```python
from build123d import *

# Parameters (mm, degrees)
SKETCH1_W           = 56
SKETCH1_H           = 56
BOSS_EXTRUDE1_DEPTH = 25
SKETCH2_W           = 53.2
SKETCH2_H           = 53.2
CUT_EXTRUDE1_DEPTH  = 22
SKETCH3_R           = 1.7
CUT_EXTRUDE2_DEPTH  = 1.4
SKETCH4_W           = 25.2
SKETCH4_H           = 27.2
CUT_EXTRUDE3_DEPTH  = 3
SKETCH5_W           = 4
SKETCH5_H           = 4
BOSS_EXTRUDE2_DEPTH = 3
SKETCH6_W           = 8
SKETCH6_H           = 8
BOSS_EXTRUDE3_DEPTH = 5
SKETCH7_R           = 2
CUT_EXTRUDE4_DEPTH  = 8
BOSS_EXTRUDE4_DEPTH = 3
FILLET1_R           = 1
CHAMFER1_SIZE       = 1.35
FILL_PATTERN1_DEPTH = 3


# Read off the part's stored shape, not the designer's step: Fill Pattern1
with BuildPart() as part:
    # Sketch1 → Boss-Extrude1 (new body)
    with BuildSketch(Plane(origin=(0, 0, 0), x_dir=(1, 0, 0), z_dir=(0, 1, 0))):
        Rectangle(SKETCH1_W, SKETCH1_H)
    extrude(amount=BOSS_EXTRUDE1_DEPTH)

    # Sketch2 → Cut-Extrude1 (cut)
    with BuildSketch(Plane(origin=(0, 25, 0), x_dir=(1, 0, 0), z_dir=(0, 1, 0))):
        Rectangle(SKETCH2_W, SKETCH2_H)
    extrude(amount=-CUT_EXTRUDE1_DEPTH, mode=Mode.SUBTRACT)

    # Sketch3 → Cut-Extrude2 (cut)
    with BuildSketch(Plane.XY.offset(28)):
        with Locations((0, 21.6)):
            Circle(SKETCH3_R)
    extrude(amount=-CUT_EXTRUDE2_DEPTH, mode=Mode.SUBTRACT)

    # Sketch4 → Cut-Extrude3 (cut)
    with BuildSketch(Plane.XZ):
        with Locations((0, 8.1)):
            Rectangle(SKETCH4_W, SKETCH4_H)
    extrude(amount=-CUT_EXTRUDE3_DEPTH, mode=Mode.SUBTRACT)

    # Sketch5 → Boss-Extrude2 (add)
    with BuildSketch(Plane.XZ):
        with Locations((-10.6, 19.7)):
            Rectangle(SKETCH5_W, SKETCH5_H)
        with Locations((10.6, 19.7)):
            Rectangle(SKETCH5_W, SKETCH5_H)
        with Locations((10.6, -3.5)):
            Rectangle(SKETCH5_W, SKETCH5_H)
        with Locations((-10.6, -3.5)):
            Rectangle(SKETCH5_W, SKETCH5_H)
    extrude(amount=-BOSS_EXTRUDE2_DEPTH)

    # Sketch6 → Boss-Extrude3 (add)
    with BuildSketch(Plane(origin=(0, 3, 0), x_dir=(1, 0, 0), z_dir=(0, 1, 0))):
        with Locations((16.6, -19.7)):
            Rectangle(SKETCH6_W, SKETCH6_H)
        with Locations((-16.6, -19.7)):
            Rectangle(SKETCH6_W, SKETCH6_H)
        Polygon((12.6, -0.5), (20.6, -0.5), (22.6, -0.5), (22.6, 9.5), (12.6, 9.5), (12.6, 7.5), align=None)
        Polygon((-12.6, -0.5), (-20.6, -0.5), (-22.6, -0.5), (-22.6, 9.5), (-12.6, 9.5), (-12.6, 7.5), align=None)
    extrude(amount=BOSS_EXTRUDE3_DEPTH)

    # Sketch7 → Cut-Extrude4 (cut)
    with BuildSketch(Plane(origin=(0, 8, 0), x_dir=(1, 0, 0), z_dir=(0, 1, 0))):
        with Locations(Location((16.6, -19.7, 0), (0, 0, 270))):
            Circle(SKETCH7_R)
        with Locations(Location((-16.6, -19.7, 0), (0, 0, 270))):
            Circle(SKETCH7_R)
        with Locations(Location((16.6, 3.5, 0), (0, 0, 270))):
            Circle(SKETCH7_R)
        with Locations(Location((-16.6, 3.5, 0), (0, 0, 270))):
            Circle(SKETCH7_R)
    extrude(amount=-CUT_EXTRUDE4_DEPTH, mode=Mode.SUBTRACT)

    # Sketch9 → Boss-Extrude4 (add)
    with BuildSketch(Plane(origin=(0, 8, 0), x_dir=(1, 0, 0), z_dir=(0, 1, 0))):
        Polygon((-22.6, -0.5), (-22.6, 9.5), (-12.6, 9.5), (-12.6, 7.65), (-20.75, 7.65), (-20.75, -0.5), align=None)
        Polygon((12.6, 9.5), (22.6, 9.5), (22.6, -0.5), (20.75, -0.5), (20.75, 7.65), (12.6, 7.65), align=None)
    extrude(amount=BOSS_EXTRUDE4_DEPTH)

    # Fillet1
    fillet1_edges = [part.edges().sort_by_distance(p)[0] for p in [
        (0, 0, 28),
        (-28, 0, 0),
        (0, 0, -28),
        (28, 0, 0),
        (28, 12.5, 28),
        (-28, 12.5, 28),
        (-28, 12.5, -28),
        (28, 12.5, -28),
    ]]
    fillet(fillet1_edges, radius=FILLET1_R)

    # Chamfer1
    chamfer1_edges = [part.edges().sort_by_distance(p)[0] for p in [
        (-1.7, 21.6, 28),
    ]]
    chamfer(chamfer1_edges, length=CHAMFER1_SIZE)

    # Fill Pattern1 outline → Fill Pattern1 (cut)
    with BuildSketch(Plane(origin=(0, 0, 0), x_dir=(1, 0, 0), z_dir=(0, 1, 0))):
        Polygon((22.516660498, 17), (24.248711306, 20), (22.516660498, 23), (19.052558883, 23), (17.320508076, 20), (19.052558883, 17), align=None)
        Polygon((8.660254038, 23), (5.196152423, 23), (3.464101615, 20), (5.196152423, 17), (8.660254038, 17), (10.392304845, 20), align=None)
        Polygon((-5.196152423, 23), (-8.660254038, 23), (-10.392304845, 20), (-8.660254038, 17), (-5.196152423, 17), (-3.464101615, 20), align=None)
        Polygon((-19.052558883, 23), (-22.516660498, 23), (-24.248711306, 20), (-22.516660498, 17), (-19.052558883, 17), (-17.320508076, 20), align=None)
        Polygon((1.732050808, 13), (3.464101615, 16), (1.732050808, 19), (-1.732050808, 19), (-3.464101615, 16), (-1.732050808, 13), align=None)
        Polygon((-12.124355653, 19), (-15.588457268, 19), (-17.320508076, 16), (-15.588457268, 13), (-12.124355653, 13), (-10.392304845, 16), align=None)
        Polygon((15.588457268, 19), (12.124355653, 19), (10.392304845, 16), (12.124355653, 13), (15.588457268, 13), (17.320508076, 16), align=None)
        Polygon((8.660254038, 9), (10.392304845, 12), (8.660254038, 15), (5.196152423, 15), (3.464101615, 12), (5.196152423, 9), align=None)
        Polygon((-5.196152423, 15), (-8.660254038, 15), (-10.392304845, 12), (-8.660254038, 9), (-5.196152423, 9), (-3.464101615, 12), align=None)
    extrude(amount=FILL_PATTERN1_DEPTH, mode=Mode.SUBTRACT)


solid = part.part
```
CAD build for the part. Positions are in the model's coordinates, mm. A direction names the side the tool comes from. Coordinates: 2 decimals unless noted, no trailing zeros. Order: outer loops, then holes, each group sorted by start corner. A loop starts at its lowest first (then second) coordinate and runs counter-clockwise, first axis right, second up.
(1) Which spindle directions (+Z, -Z, +X, -X, +Y, -Y) get a long thin tool onto all of the face, cutting with end or side? Do faces 1 (the face through (-23.37, 1.48, -21.52)), 2 (the face through (-18, 8, 18)). Say none if no direction does.
Solution:
face 1: +Y, -Y
face 2: +Y
(2) Saw through at A-A, the plane y = 7.25. Count the separate pieces of the cut face and the enclosed holes in it, and give its area (3 significant figures).
Solution:
separate pieces: 5
enclosed holes: 5
area: 583 mm2
(3) Saw through at C-C, the plane x = 0. Write the cut outline in (y, z), and give its area (3 significant figures).
Solution:
outline: (0, -27) arc R1 ccw to (1, -28) - (25, -28) - (25, -26.6) - (3, -26.6) - (3, -19) - (0, -19) - close; (0, -13) - (3, -13) - (3, -5.5) - (0, -5.5) - close; (0, 21.7) - (3, 21.7) - (3, 26.6) - (19.9, 26.6) - (19.9, 26.65) - (18.55, 28) - (1, 28) arc R1 ccw to (0, 27) - close; (23.3, 26.6) - (25, 26.6) - (25, 28) - (24.65, 28) - (23.3, 26.65) - close
area: 123 mm2
(4) Pin check, flat tip, straight feed: pin 1 Ø2.5 at (x, z) = (15, -2) entering from +Y. Stop position of the tip, or through.
Solution:
pin 1: stops at y = 8
(5) Drill centre lines: L1, parallel to X at y = 6.75, z = 19.7; L2, parallel to X at y = 8.75, z = -1; L3, parallel to X at y = 4, z = -3.5. Where is each one in solid material? Low to high.
Solution:
L1: x = -28 to -26.6, -20.6 to -18.6, -14.6 to -12.6, 12.6 to 14.6, 18.6 to 20.6, 26.6 to 28
L2: x = -28 to -26.6, -22.6 to -20.75, 20.75 to 22.6, 26.6 to 28
L3: x = -28 to -26.6, -22.6 to -18.6, -14.6 to -12.6, 12.6 to 14.6, 18.6 to 22.6, 26.6 to 28
(6) Mould opens along X. For faces 3 (the face through (17, 5, 23.7)), 4 (the face through (-2, 25, 27)) say: released by +X, released by -X, zero draft, split by the parting line, or undercut.
Solution:
face 3: undercut
face 4: zero draft
(7) Saw through at D-D, the plane y = 14.5. Write the cut outline in (x, z).
Solution:
outline: (-28, -27) arc R1 ccw to (-27, -28) - (27, -28) arc R1 ccw to (28, -27) - (28, 27) arc R1 ccw to (27, 28) - (-27, 28) arc R1 ccw to (-28, 27) - close; hole (-26.6, -26.6) - (26.6, -26.6) - (26.6, 26.6) - (-26.6, 26.6) - close
